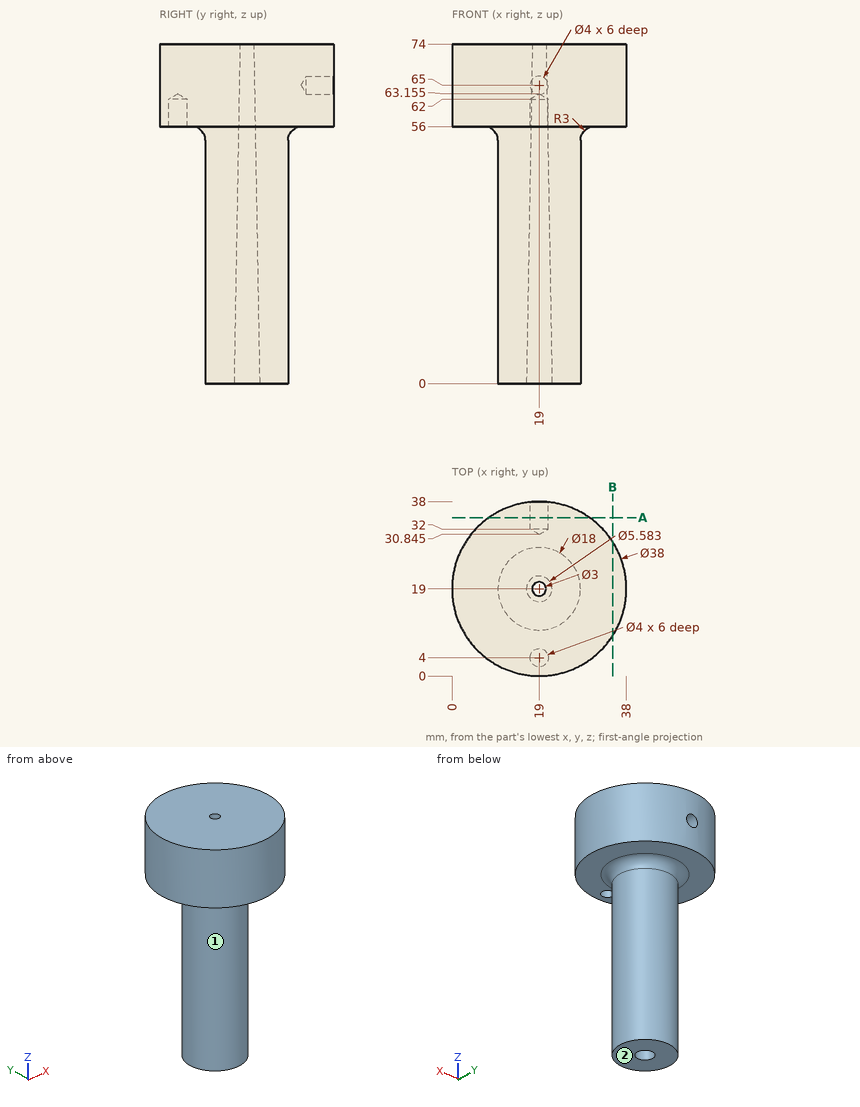
Drawing for the job (mm, zero at the part's lowest x, y, z). A direction names the side the tool comes from. Give positions to 0.01 mm unless a question says otherwise; leave off trailing zeros. Order: outer loops, then holes, each group sorted by start corner. A loop starts at its lowest first (then second) coordinate and runs counter-clockwise, first axis right, second up. Notation, with made-up numbers: M 83.25,-11 L 133.25,-11 A18 cw 133.25,20 Z; hole C 35.5,45 d2. An arc over 180 degrees is marked long. Use a Markdown table: item, result. Add a question column.
(1) Drop flat-ended pins along their axis: P1, Ø8, axis at y = 11, z = 13.5, coming from the -X side; P2, Ø2, axis at y = 11, z = 56, coming from the +X side; P3, Ø3, axis at y = 12, z = 31.5, coming from the -X side (1 decimal). Give the stop position or say it passes through.
(2) Probe line 1 along Y through (x, z) = (18.5, 59); line 2 along Y through (x, z) = (19, 57.75); line 3 along Y through (x, z) = (19, 37.5). List the from-to ranges inside material, lowest first. Write a range as [from, to].
(3) 3-axis set-ups, long thin cutter, end or side, ignore diameter. For the marked faces 1 and 2: which of +Z, -Z, +X, -X, +Y, -Y reach the whole face in a straight line?
(4) Saw through at A-A, the plane y = 34.5. Give the cut face in (x, z), and give its area (3 significant figures).
(5) Saw through at B-B, the plane x = 35. Give the cut face in (y, z), and give its area (3 significant figures).
Answer key:
| question | item | result |
|---|---|---|
| 1 | P1 | x = 10.94 |
| 1 | P2 | x = 36.66 |
| 1 | P3 | x = 11.9 |
| 2 | line 1 | [0.01, 2.06], [5.94, 17.31], [20.69, 37.99] |
| 2 | line 2 | [0, 2], [6, 17.22], [20.78, 38] |
| 2 | line 3 | [10, 16.86], [21.14, 28] |
| 3 | face 1 | -Z |
| 3 | face 2 | -Z, +X, -X, +Y, -Y |
| 4 | outline | M 8.01,56 L 29.99,56 L 29.99,74 L 8.01,74 Z; hole C 19,65 d4 |
| 4 | area | 383 mm^2 |
| 5 | outline | M 8.75,56 L 29.25,56 L 29.25,74 L 8.75,74 Z |
| 5 | area | 369 mm^2 |
